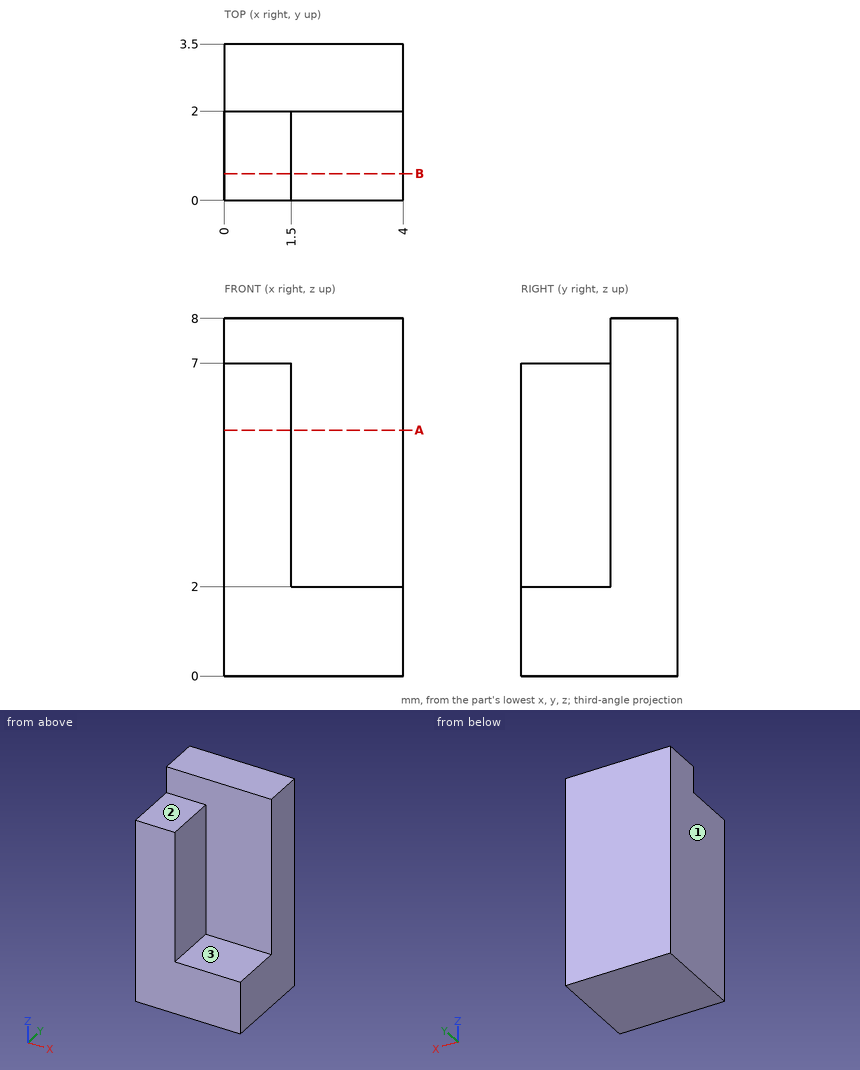
The figure shows three views and two pictorial views of one solid part (mm, origin at its lowest corner). Answer the questions. A direction names the side the tool comes from. Round coordinates to 2 decimals unless told otherwise and drop trailing zeros. Write each loop counter-clockwise with the first axis right and the second up, starting at its lowest first coordinate (ties: lowest second). Pieces come first, ordered by that corner, then holes. Notation, with made-up numbers: (-11, -10) - (17, -10) arc R25 cw to (17, 10) - close; hole circle Ø8 at (-15, 77.25). An arc over 180 degrees is marked (long way). Answer in a Markdown table with one row per item. Add a question column.
1. A cutting plane is placed at A-A, the plane z = 5.5. Determine the outline of the cut face in (x, y), and give its area (3 significant figures).
2. Given pin 1 (2 mm diameter, centred on x = 1, z = 6, fed in from -Y); pin 2 (1 mm diameter, centred on y = 1, z = 5.5, fed in from +X); pin 3 (1.2 mm diameter, centred on x = 1, y = 1, fed in from +Z); pin 4 (1 mm diameter, centred on x = 3.5, z = 5, fed in from -Y), each flat-ended and moving along its own axis, determine where each tip first touches the part or whether it passes through.
3. A cutting plane is placed at B-B, the plane y = 0.6. Determine the outline of the cut face in (x, z), and give its area (3 significant figures).
4. For the marked faces 1, 2 and 3, determine the directions among +Z, -Z, +X, -X, +Y, -Y from which every point of the face is accessible in a straight line to the end or side of a thin tool.
5. Find the intervals of material crossed by line 1 along Z through (x, y) = (1.65, 1.7); line 2 along Y through (x, z) = (2.5, 7.5); line 3 along Z through (x, y) = (0.7, 1.5), in increasing order. Write a range as from..to.
Worked out:
| question | item | result |
|---|---|---|
| 1 | outline | (0, 0) - (1.5, 0) - (1.5, 2) - (4, 2) - (4, 3.5) - (0, 3.5) - close |
| 1 | area | 9.00 mm^2 |
| 2 | pin 1 | y = 0 |
| 2 | pin 2 | x = 1.5 |
| 2 | pin 3 | z = 7 |
| 2 | pin 4 | y = 2 |
| 3 | outline | (0, 0) - (4, 0) - (4, 2) - (1.5, 2) - (1.5, 7) - (0, 7) - close |
| 3 | area | 15.5 mm^2 |
| 4 | face 1 | +Z, -Z, -X, +Y, -Y |
| 4 | face 2 | +Z, +X, -X, -Y |
| 4 | face 3 | +Z, +X, -Y |
| 5 | line 1 | 0..2 |
| 5 | line 2 | 2..3.5 |
| 5 | line 3 | 0..7 |
